The drawing under review shows one solid part. Ordinate dimensions are in mm from its lowest x, y, z. A direction names the side the tool comes from. Coordinates: 2 decimals unless noted, no trailing zeros. Write each loop counter-clockwise with the first axis right and the second up, starting at its lowest first coordinate (ties: lowest second). Pieces come first, ordered by that corner, then holes.
1) For P1, Ø5, axis at y = 75.5, z = 66, coming from the +X side; P2, Ø6, axis at x = 90.5, z = 14, coming from the -Y side; P3, Ø12, axis at x = 178.5, y = 136, coming from the +Z side, all flat-tipped, find the tip position at first contact; note any pin that passes through.
2) Add section A-A, the plane y = 301.5. State the section outline as (x, z) points.
3) Add section D-D, the plane x = 249. State the section outline as (y, z) points.
4) Machinability: for the marked faces 1 and 2, which of the approach directions +Z, -Z, +X, -X, +Y, -Y give a long, thin tool a straight path to every point of the face, cutting with its end or side? Answer none if there is none.
5) For line 1 (Y direction, x = 206.5, z = 18); line 2 (Y direction, x = 260, z = 12); line 3 (X direction, y = 234, z = 10), list the stretches that pass through material, from the lowest coordinate up.
6) Add section B-B, the plane x = 339.5. State the section outline as (y, z) points.
7) Add section C-C, the plane z = 14.5. State the section outline as (x, y) points.
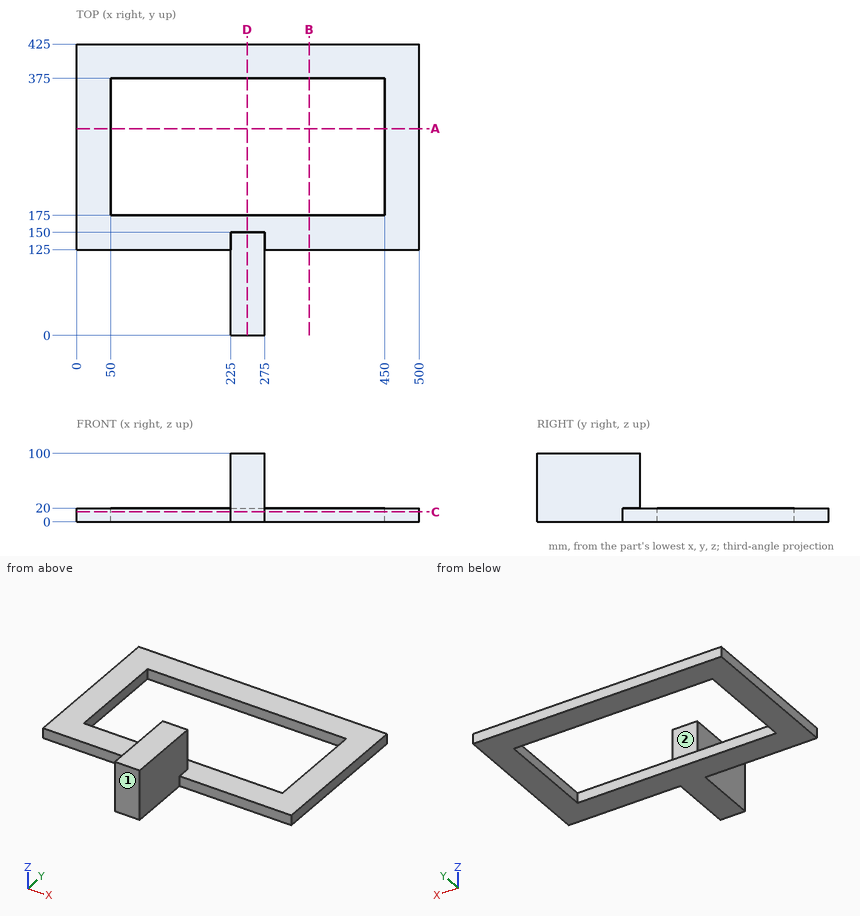
Geometry results:
1. P1: stops at x = 275
1. P2: stops at y = 125
1. P3: stops at z = 20
2. outline: (0, 0) - (50, 0) - (50, 20) - (0, 20) - close; (450, 0) - (500, 0) - (500, 20) - (450, 20) - close
3. outline: (0, 0) - (175, 0) - (175, 20) - (150, 20) - (150, 100) - (0, 100) - close; (375, 0) - (425, 0) - (425, 20) - (375, 20) - close
4. face 1: +Z, -Z, +X, -X, -Y
4. face 2: +Z, +X, -X, +Y
5. line 1: y = 125 to 175, 375 to 425
5. line 2: y = 0 to 175, 375 to 425
5. line 3: x = 0 to 50, 450 to 500
6. outline: (125, 0) - (175, 0) - (175, 20) - (125, 20) - close; (375, 0) - (425, 0) - (425, 20) - (375, 20) - close
7. outline: (0, 125) - (225, 125) - (225, 0) - (275, 0) - (275, 125) - (500, 125) - (500, 425) - (0, 425) - close; hole (50, 175) - (450, 175) - (450, 375) - (50, 375) - close
